```python
from build123d import *

# Parameters (mm, degrees)
SKETCH1_R               = 20
SKETCH1_R_2             = 6
SKETCH1_R_3             = 2.25
BOSS_EXTRUDE1_DEPTH     = 4.6
CUT_EXTRUDE1_DEPTH      = 29.655889447
CUT_EXTRUDE1_DEPTH_BACK = 29.655889447
SKETCH2_R               = 2.25
FILLET2_R               = 5


with BuildPart() as part:
    # Sketch1 → Boss-Extrude1 (new body)
    with BuildSketch(Plane(origin=(0, 0, 0), x_dir=(1, 0, 0), z_dir=(0, 1, 0))):
        with Locations(Location((0, 0, 0), (0, 0, 270))):
            Circle(SKETCH1_R)
        with Locations(Location((0, 0, 0), (0, 0, 270))):
            Circle(SKETCH1_R_2, mode=Mode.SUBTRACT)
        with Locations(Location((0, 12.5, 0), (0, 0, 270))):
            Circle(SKETCH1_R_3, mode=Mode.SUBTRACT)
        with Locations(Location((10.825317547, 6.25, 0), (0, 0, 270))):
            Circle(SKETCH1_R_3, mode=Mode.SUBTRACT)
        with Locations(Location((10.825317547, -6.25, 0), (0, 0, 270))):
            Circle(SKETCH1_R_3, mode=Mode.SUBTRACT)
        with Locations(Location((0, -12.5, 0), (0, 0, 270))):
            Circle(SKETCH1_R_3, mode=Mode.SUBTRACT)
        with Locations(Location((-10.825317547, -6.25, 0), (0, 0, 270))):
            Circle(SKETCH1_R_3, mode=Mode.SUBTRACT)
        with Locations(Location((-10.825317547, 6.25, 0), (0, 0, 270))):
            Circle(SKETCH1_R_3, mode=Mode.SUBTRACT)
    extrude(amount=BOSS_EXTRUDE1_DEPTH)

    # Sketch2 → Cut-Extrude1 (cut, two sides: drawn at the far end of the back side and taken through both)
    with BuildSketch(Plane(origin=(0, 4.6, 0), x_dir=(1, 0, 0), z_dir=(0, 1, 0)).offset(-CUT_EXTRUDE1_DEPTH_BACK)):
        with BuildLine():
            Line((13.599697882, 14.66452241), (-2.005277819, 5.654985488))
            ThreePointArc((-2.005277819, 5.654985488), (3.461815498, 4.900595214), (6, 0))
            ThreePointArc((6, 0), (5.448317772, -2.5131322), (3.894722181, -4.564114277))
            Line((3.894722181, -4.564114277), (19.499697882, 4.445422645))
            ThreePointArc((19.499697882, 4.445422645), (17.320508076, 10), (13.599697882, 14.66452241))
        make_face()
        with Locations((10.825317547, 6.25)):
            Circle(SKETCH2_R, mode=Mode.SUBTRACT)
    extrude(amount=CUT_EXTRUDE1_DEPTH + CUT_EXTRUDE1_DEPTH_BACK, mode=Mode.SUBTRACT)

    # Fillet2
    fillet2_edges = [part.edges().sort_by_distance(p)[0] for p in [
        (19.499697882, 2.3, -4.445422645),
        (13.599697882, 2.3, -14.66452241),
    ]]
    fillet(fillet2_edges, radius=FILLET2_R)


solid = part.part
```
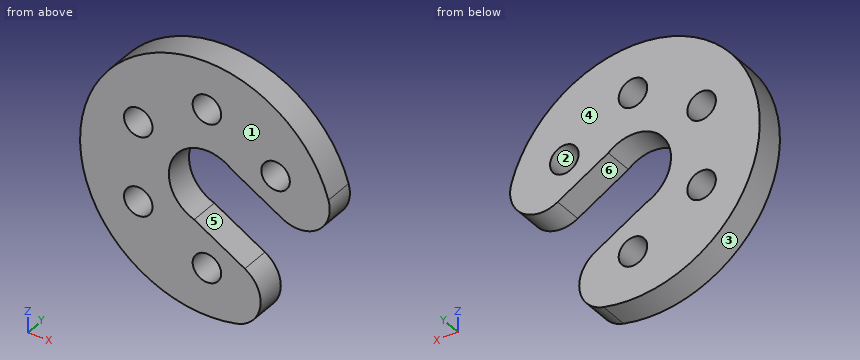
Input: part model. Units: mm. Frame: model coordinates. Face numbers are marked on the shaded views. A direction names the side the tool comes from. Coordinates: 2 decimals unless noted, no trailing zeros. Loops run counter-clockwise (first coordinate to the right, second up) from the corner with the lowest first, then second, coordinate; pieces in that order, holes last. Notation, with made-up numbers: M 57.25,32 L 96.25,32 A26 ccw 96.25,51 Z; hole C 41.5,-13.75 d5. An arc over 180 degrees is marked long. Answer in a Markdown table with one row per item.
1. Draft query along Z for the marked faces 1, 2 and 3. Return one class per face: pulls with the +Z half, pulls with the -Z half, needs draft (parallel to the pull), parting line crosses it, or undercut.
Response:
| item | result |
|---|---|
| face 1 | needs draft |
| face 2 | undercut |
| face 3 | parting line crosses it |
2. Material intervals for line 1 (X direction, y = 1.85, z = 6.25); line 2 (X direction, y = 0.4, z = 6.5); line 3 (X direction, y = 1.3, z = 5), sorted ascending.
Response:
| item | result |
|---|---|
| line 1 | x = -19 to -13.08, -8.58 to 8.58, 13.08 to 19 |
| line 2 | x = -18.91 to -13.06, -8.59 to 8.59, 13.06 to 18.91 |
| line 3 | x = -19.36 to -12.7, -8.95 to -3.32, 3.32 to 8.95, 12.7 to 19.32 |
3. Reachability of the marked faces 4, 5 and 6 from +Z, -Z, +X, -X, +Y, -Y: full face, straight path, thin tool, end or side. Return the list, or none.
Response:
| item | result |
|---|---|
| face 4 | +Z, -Z, +X, -X, +Y |
| face 5 | +X, +Y, -Y |
| face 6 | +Y, -Y |
4. Section B-B, the plane x = 8. Output: boundary loops of the cut face in (y, z).
Response:
| item | result |
|---|---|
| outline | M 0,-16.72 L 4.6,-16.72 L 4.6,-12.47 L 0,-12.47 Z; M 0,2.19 L 4.6,2.19 L 4.6,18.33 L 0,18.33 Z |
5. Section A-A, the plane z = -8. Output: boundary loops of the cut face in (x, y).
Response:
| item | result |
|---|---|
| outline | M -18.33,0 L -12.24,0 L -12.24,4.6 L -18.33,4.6 Z; M -9.41,0 L 2.06,0 L 2.06,4.6 L -9.41,4.6 Z |
6. Section D-D, the plane x = -15.5. Output: boundary loops of the cut face in (y, z).
Response:
| item | result |
|---|---|
| outline | M 0,-12.64 L 4.6,-12.64 L 4.6,12.64 L 0,12.64 Z |
7. Section C-C, the plane y = 0.9. Output: boundary loops of the cut face in (x, z).
Response:
| item | result |
|---|---|
| outline | M -2.01,-5.65 A6 cw long 3.89,4.56 L 11.87,-0.04 A5 ccw 19.17,5.72 A20 ccw long 4.63,-19.46 A5 ccw 5.97,-10.26 Z; hole C -10.83,-6.25 d4.5; hole C -10.83,6.25 d4.5; hole C 0,-12.5 d4.5; hole C 0,12.5 d4.5; hole C 10.83,6.25 d4.5 |
